Model file for the job. Use its own axes, mm. Coordinates: 2 decimals unless noted, no trailing zeros. Write each loop counter-clockwise with the first axis right and the second up, starting at its lowest first coordinate (ties: lowest second). Pieces come first, ordered by that corner, then holes. Notation, with made-up numbers: M 72,73.5 L 89,73.5 A20 cw 89,83.5 Z; hole C 30.5,74 d6. An arc over 180 degrees is marked long. Put each result on its own line as item: value. Start each with the question number.
Q1. Pull direction X, two halves, no side cores. Call faces 1 (the cylindrical face through (-6.6, -29.723, 25.044)), 2 (the flat face through (53.469, 26.533, 25.044)), 3 (the flat face through (31, 1, 0)), 4 (the cylindrical face through (-46.76, -1.41, 25.04)): pulls with the +X half, pulls with the -X half, needs draft (parallel to the pull), parting line crosses it, or undercut.
Q2. Cut at C-C (y = -6). Write the cut outline in (x, z).
Q3. Cut at B-B (z = 5.5). Write the cut outline in (x, y).
Q4. Drop flat-ended pins along their axis: pin 1 (6 mm diameter, centred on y = 29.5, z = 9.5, fed in from -X); pin 2 (6 mm diameter, centred on y = 15, z = 43, fed in from +X); pin 3 (12 mm diameter, centred on y = 37, z = 14.5, fed in from -X). Give the stop position or say it passes through.
Q5. Drill centre lines: line 1 along Y through (x, z) = (0, 36.5); line 2 along X through (y, z) = (-26, 20); line 3 along Y through (x, z) = (-27, 29). Where is each one in solid material? Low to high.
Q6. Cut at D-D (y = 36.5). Write the cut outline in (x, z), then the cut area to 3 significant figures.
Q7. Cut at A-A (x = 0). Write the cut outline in (y, z), then the cut area to 3 significant figures.
```python
from build123d import *

# Parameters (mm, degrees)
F0_R     = 30.447507
F1_DEPTH = 50.8


with BuildPart() as f1:
    # F0 (on Top) → F1 (new body)
    with BuildSketch(Plane.XY):
        Circle(F0_R)
        with BuildLine():
            ThreePointArc((22.158063, -41.202629), (40.157528, -24.000195), (46.782864, 0))
            ThreePointArc((46.782864, 0), (40.969486, 22.586226), (24.974127, 39.559188))
            Line((24.974127, 39.559188), (13.576085, 44.769703))
            ThreePointArc((13.576085, 44.769703), (-46.706625, -2.669747), (18.589059, -42.931146))
            Line((18.589059, -42.931146), (22.158063, -41.202629))
        make_face()
        Circle(F0_R, mode=Mode.SUBTRACT)
        with BuildLine():
            ThreePointArc((24.974127, 39.559188), (40.969486, 22.586226), (46.782864, 0))
            Line((46.782864, 0), (81.176508, 0))
            Line((81.176508, 0), (81.176508, 13.866764))
            Line((81.176508, 13.866764), (24.974127, 39.559188))
        make_face()
        with BuildLine():
            Line((81.176508, 0), (46.782864, 0))
            ThreePointArc((46.782864, 0), (40.157528, -24.000195), (22.158063, -41.202629))
            Line((22.158063, -41.202629), (81.176508, -12.619201))
            Line((81.176508, -12.619201), (81.176508, 0))
        make_face()
        with BuildLine():
            Line((13.576085, 44.769703), (24.974127, 39.559188))
            ThreePointArc((24.974127, 39.559188), (19.450375, 42.547848), (13.576085, 44.769703))
        make_face()
        with BuildLine():
            ThreePointArc((18.589059, -42.931146), (20.391884, -42.104721), (22.158063, -41.202629))
            Line((22.158063, -41.202629), (18.589059, -42.931146))
        make_face()
        Polygon((81.176508, 13.866764), (81.176508, 0), (111.018896, 0), align=None)
        Polygon((111.018896, 0), (81.176508, 0), (81.176508, -12.619201), align=None)
    extrude(amount=F1_DEPTH)


solid = f1.part
```
Computed values:
1. face 1: undercut
1. face 2: pulls with the +X half
1. face 3: needs draft
1. face 4: parting line crosses it
2. outline: M -46.4,0 L -29.85,0 L -29.85,50.8 L -46.4,50.8 Z; M 29.85,0 L 96.83,0 L 96.83,50.8 L 29.85,50.8 Z
3. outline: M 13.58,44.77 A46.78 ccw long 18.59,-42.93 A46.78 ccw 22.16,-41.2 L 81.18,-12.62 L 111.02,0 L 81.18,13.87 L 24.97,39.56 A46.78 ccw Z; hole C 0,0 d60.9
4. pin 1: x = -38.55
4. pin 2: x = 85.19
4. pin 3: x = -35.04
5. line 1: -46.78 to -30.45, 30.45 to 46.78
5. line 2: -38.89 to -15.84, 15.84 to 53.55
5. line 3: -38.21 to -14.07, 14.07 to 38.21
6. outline: M -29.26,0 L 31.67,0 L 31.67,50.8 L -29.26,50.8 Z
6. area: 3,100 mm2
7. outline: M -46.78,0 L -30.45,0 L -30.45,50.8 L -46.78,50.8 Z; M 30.45,0 L 46.78,0 L 46.78,50.8 L 30.45,50.8 Z
7. area: 1,660 mm2
